Check sheet for the modelled part. Datum: model origin and axes. Units: mm. A direction names the side the tool comes from. Round coordinates to 2 decimals unless told otherwise and drop trailing zeros. Order: outer loops, then holes, each group sorted by start corner. A loop starts at its lowest first (then second) coordinate and runs counter-clockwise, first axis right, second up.
```python
from build123d import *

# Parameters (mm, degrees)
SKETCH_1_R           = 4
SKETCH_1_R_2         = 1.7
EXTRUDE_1_DEPTH      = 6
EXTRUDE_2_DEPTH      = 2
EXTRUDE_2_DEPTH_BACK = 2
SKETCH_3_R           = 1.75
EXTRUDE_3_DEPTH      = 2.8
EXTRUDE_3_DEPTH_BACK = 2.8


with BuildPart() as part:
    # Sketch 1 → Extrude 1 (new body)
    with BuildSketch(Plane.XY):
        Circle(SKETCH_1_R)
        Circle(SKETCH_1_R_2, mode=Mode.SUBTRACT)
    extrude_1 = extrude(amount=EXTRUDE_1_DEPTH)

    # Sketch 2 → Extrude 2 (add, two sides)
    with BuildSketch(Plane(origin=(0, 0, 0), x_dir=(1, 0, 0), z_dir=(0, 1, 0))) as extrude_2_sk:
        Polygon((-4, 0), (-12, -6), (-12, -12.6), (-4, -18.6), (-3, -18.6), (-3, -12.6), (-4, -12.6), (-6.5, -12.6), (-6.5, -6), (-4, -6), (-3.5, -6), (-3.5, 0), align=None)
    extrude(amount=EXTRUDE_2_DEPTH)
    extrude(extrude_2_sk.sketch, amount=-EXTRUDE_2_DEPTH_BACK)

    # Mirror 1: Extrude 1 across plane
    add(extrude_1.mirror(Plane(origin=(0, 0, 9.3), x_dir=(1, 0, 0), z_dir=(0, 0, -1))))

    # Sketch 3 → Extrude 3 (add, two sides)
    with BuildSketch(Plane(origin=(0, 0, 9.3), x_dir=(-1, 0, 0), z_dir=(0, 0, -1))) as extrude_3_sk:
        with BuildLine():
            Line((19.5, 4), (24.5, 4))
            ThreePointArc((24.5, 4), (26.5, 3.464101615), (27.964101615, 2))
            Line((27.964101615, 2), (30.035898385, 2))
            ThreePointArc((30.035898385, 2), (37.5, 0), (30.035898385, -2))
            Line((30.035898385, -2), (27.964101615, -2))
            ThreePointArc((27.964101615, -2), (26.5, -3.464101615), (24.5, -4))
            Line((24.5, -4), (19.5, -4))
            ThreePointArc((19.5, -4), (17.5, -3.464101615), (16.035898385, -2))
            Line((16.035898385, -2), (12, -2))
            Line((12, -2), (12, 2))
            Line((12, 2), (16.035898385, 2))
            ThreePointArc((16.035898385, 2), (17.5, 3.464101615), (19.5, 4))
        make_face()
        with Locations((33.5, 0)):
            Circle(SKETCH_3_R, mode=Mode.SUBTRACT)
        with BuildLine():
            Line((19.5, 1.8), (24.5, 1.8))
            ThreePointArc((24.5, 1.8), (26.3, 0), (24.5, -1.8))
            Line((24.5, -1.8), (19.5, -1.8))
            ThreePointArc((19.5, -1.8), (17.7, 0), (19.5, 1.8))
        make_face(mode=Mode.SUBTRACT)
    extrude(amount=EXTRUDE_3_DEPTH)
    extrude(extrude_3_sk.sketch, amount=-EXTRUDE_3_DEPTH_BACK)


solid = part.part
```
Item 1: Sectioned sample at A-A (x = 0). Record the cut outline in (y, z).
Answer:
outline: (-4, 0) - (-1.7, 0) - (-1.7, 6) - (-4, 6) - close; (-4, 12.6) - (-1.7, 12.6) - (-1.7, 18.6) - (-4, 18.6) - close; (1.7, 0) - (4, 0) - (4, 6) - (1.7, 6) - close; (1.7, 12.6) - (4, 12.6) - (4, 18.6) - (1.7, 18.6) - close
Item 2: Sectioned sample at B-B (z = 8.5). Record the cut outline in (x, y), and give its area (3 significant figures).
Answer:
outline: (-30.04, -2) - (-27.96, -2) arc R4 ccw to (-24.5, -4) - (-19.5, -4) arc R4 ccw to (-16.04, -2) - (-6.5, -2) - (-6.5, 2) - (-16.04, 2) arc R4 ccw to (-19.5, 4) - (-24.5, 4) arc R4 ccw to (-27.96, 2) - (-30.04, 2) arc R4 ccw (long way) to start; hole circle Ø3.5 at (-33.5, 0); hole (-24.5, -1.8) - (-19.5, -1.8) arc R1.8 ccw to (-19.5, 1.8) - (-24.5, 1.8) arc R1.8 ccw to start
area: 145 mm2
Item 3: Go/stop test with flat-tipped pins: P1, Ø2.5, axis at x = -29.5, z = 9.5, coming from the -Y side; P2, Ø10, axis at x = -10, z = 9, coming from the +Y side; P3, Ø2, axis at x = 0, y = 0, coming from the +Z side; P4, Ø1, axis at x = -13.5, y = -1, coming from the -Z side. Record where each tip stops, or that it passes through.
Answer:
P1: stops at y = -2.9
P2: stops at y = 2
P3: passes through
P4: stops at z = 6.5
Item 4: Sectioned sample at C-C (y = 0). State how many separate pieces and enclosed holes the cut face has, and give its area (3 significant figures).
Answer:
separate pieces: 5
enclosed holes: 0
area: 215 mm2
Item 5: Access from +Z, -Z, +X, -X, +Y, -Y to the whole of each face (thin tool, end or side, straight path). Record for faces 1 (the flat face through (-22, -1.8, 9)), 2 (the flat face through (-25, 2, 6.5)), 3 (the flat face through (-25, 2, 12.1)), 4 (the flat face through (-2, 0, 12.6)), 5 (the flat face through (-29, 2, 9)).
Answer:
face 1: +Z, -Z
face 2: -Z, -X, +Y, -Y
face 3: +Z, -X, +Y, -Y
face 4: +X, +Y, -Y
face 5: +Z, -Z, +Y
Item 6: Sectioned sample at D-D (x = -21.5). Record the cut outline in (y, z), and give its area (3 significant figures).
Answer:
outline: (-4, 6.5) - (-1.8, 6.5) - (-1.8, 12.1) - (-4, 12.1) - close; (1.8, 6.5) - (4, 6.5) - (4, 12.1) - (1.8, 12.1) - close
area: 24.6 mm2
Item 7: Scan lines: line 1 along Y through (x, z) = (0, 4.65); line 2 along Z through (x, y) = (-1, 3.25); line 3 along X through (y, z) = (0.75, 11). Record each from-to range of solid material in increasing order.
Answer:
line 1: y = -4 to -1.7, 1.7 to 4
line 2: z = 0 to 6, 12.6 to 18.6
line 3: x = -37.43 to -35.08, -31.92 to -26.14, -17.86 to -6.5
Item 8: Release check for a two-part mould opening along Z. For faces 6 (the flat face through (-6.5, 0, 9)), 7 (the flat face through (-22, -4, 9)), 8 (the flat face through (0, -2, 18.6)) record: released by +Z, released by -Z, zero draft, split by the parting line, or undercut.
Answer:
face 6: undercut
face 7: zero draft
face 8: released by +Z
